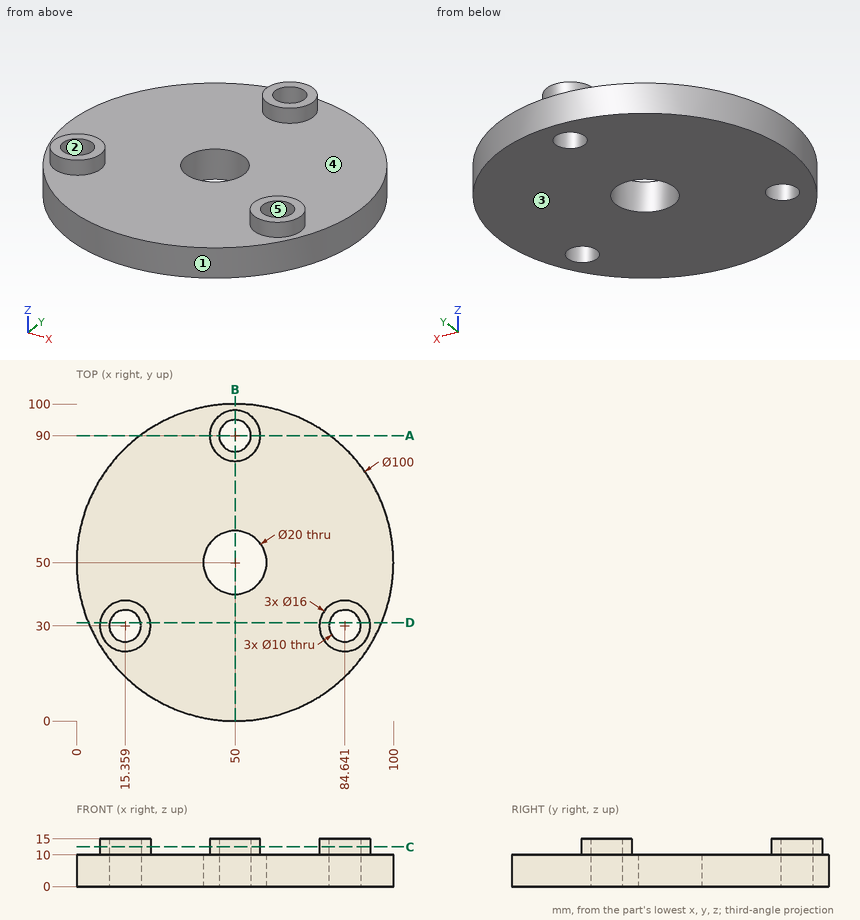
Check sheet for the drawn part. Datum: minimum x, y, z corner. Units: mm. A direction names the side the tool comes from. Give positions to 0.01 mm unless a question says otherwise; leave off trailing zeros. Write each loop counter-clockwise with the first axis right and the second up, starting at its lowest first coordinate (ties: lowest second). Pieces come first, ordered by that corner, then holes. Notation, with made-up numbers: (29.5, 14) -> (74.5, 14) arc R25 cw to (74.5, 42) -> close; hole circle Ø2 at (81.25, 87.5). An arc over 180 degrees is marked (long way). Use one line per item in the form item = value. Start each with the question number.
1. Thickness scan on line 1 along Y through (x, z) = (50, 6.5); line 2 along X through (y, z) = (27.5, 4.25); line 3 along Z through (x, y) = (11.5, 70). Record the ranges inside material, lowest first. Write a range as from..to.
2. Section check D-D (y = 31). Record the cut outline in (x, z).
3. Go/stop test with flat-tipped pins: P1, Ø3, axis at x = 47.5, z = 12, coming from the +Y side; P2, Ø13, axis at x = 84.64, y = 30, coming from the -Z side; P3, Ø16, axis at x = 50, y = 50, coming from the +Z side; P4, Ø1, axis at x = 88.5, z = 7.5, coming from the +Y side. Record where each tip stops, or that it passes through.
4. Mould release check, pull along Y, two halves, no side actions. Record for the marked faces 1, 2 and 3: pulls with the +Y half, pulls with the -Y half, needs draft (parallel to the pull), parting line crosses it, or undercut.
5. Section check A-A (y = 90). Record the cut outline in (x, z), and give its area (3 significant figures).
6. Section check C-C (z = 12.5). Record the cut outline in (x, y), and give its area (3 significant figures).
7. Section check B-B (x = 50). Record the cut outline in (y, z).
8. Access from +Z, -Z, +X, -X, +Y, -Y to the whole of each face (thin tool, end or side, straight path). Record for the marked faces 4 and 5.
Conclusion:
q1.line_1 = 0..40, 60..85, 95..100
q1.line_2 = 5.35..11.03, 19.69..80.31, 88.97..94.65
q1.line_3 = 0..10
q2.outline = (3.75, 0) -> (10.46, 0) -> (10.46, 15) -> (7.42, 15) -> (7.42, 10) -> (3.75, 10) -> close; (20.26, 0) -> (79.74, 0) -> (79.74, 15) -> (76.7, 15) -> (76.7, 10) -> (23.3, 10) -> (23.3, 15) -> (20.26, 15) -> close; (89.54, 0) -> (96.25, 0) -> (96.25, 10) -> (92.58, 10) -> (92.58, 15) -> (89.54, 15) -> close
q3.P1 = 97.94
q3.P2 = 0
q3.P3 = through
q3.P4 = 82.5
q4.face_1 = parting line crosses it
q4.face_2 = undercut
q4.face_3 = needs draft
q5.outline = (20, 0) -> (45, 0) -> (45, 15) -> (42, 15) -> (42, 10) -> (20, 10) -> close; (55, 0) -> (80, 0) -> (80, 10) -> (58, 10) -> (58, 15) -> (55, 15) -> close
q5.area = 530 mm²
q6.outline = circle Ø16 at (15.36, 30); circle Ø16 at (50, 90); circle Ø16 at (84.64, 30); hole circle Ø10 at (15.36, 30); hole circle Ø10 at (50, 90); hole circle Ø10 at (84.64, 30)
q6.area = 368 mm²
q7.outline = (0, 0) -> (40, 0) -> (40, 10) -> (0, 10) -> close; (60, 0) -> (85, 0) -> (85, 15) -> (82, 15) -> (82, 10) -> (60, 10) -> close; (95, 0) -> (100, 0) -> (100, 10) -> (98, 10) -> (98, 15) -> (95, 15) -> close
q8.face_4 = +Z
q8.face_5 = +Z, -Z
